```python
from build123d import *

# Parameters (mm, degrees)
F0_W        = 98
F0_H        = 136
F0_W_2      = 78
F0_H_2      = 116
F0_W_3      = 75
F0_H_3      = 113
F1_DEPTH    = 5
F2_W        = 78
F2_H        = 130
F3_DEPTH    = 0.5
F5_T1_DEPTH = 85
F6_R        = 5


# Not quite as in the source:
# - a fillet or chamfer that OpenCascade refuses, or shapes differently, is made with other operations: its cross-section is extruded or revolved along the edge and cut away or added
# - a feature of the source that left no trace in its solid (it failed there, or was rolled back) is left out


with BuildPart() as f1:
    # F0 (on Top) → F1 (new body, symmetric)
    with BuildSketch(Plane.XY):
        Rectangle(F0_W, F0_H)
        Rectangle(F0_W_2, F0_H_2, mode=Mode.SUBTRACT)
        Rectangle(F0_W_2, F0_H_2)
        Rectangle(F0_W_3, F0_H_3, mode=Mode.SUBTRACT)
    extrude(amount=F1_DEPTH, both=True)

    # F2 (on Top) → F3 (cut, symmetric)
    with BuildSketch(Plane.XY):
        with Locations((0, 7)):
            Rectangle(F2_W, F2_H)
    extrude(amount=F3_DEPTH, both=True, mode=Mode.SUBTRACT)

    # F5: fillet of radius 15 on 4 edges, made by hand

    # F5_s2 → F5_t1 (cut)
    with BuildSketch(Plane.XY.offset(-42.5)):
        with BuildLine():
            ThreePointArc((-34, -68), (-44.6066017178, -63.6066017178), (-49, -53))
            Line((-49, -53), (-49, -68))
            Line((-49, -68), (-34, -68))
        make_face()
        with BuildLine():
            ThreePointArc((34, -68), (44.6066017178, -63.6066017178), (49, -53))
            Line((49, -53), (49, -68))
            Line((49, -68), (34, -68))
        make_face()
        with BuildLine():
            ThreePointArc((34, 68), (44.6066017178, 63.6066017178), (49, 53))
            Line((49, 53), (49, 68))
            Line((49, 68), (34, 68))
        make_face()
        with BuildLine():
            ThreePointArc((-34, 68), (-44.6066017178, 63.6066017178), (-49, 53))
            Line((-49, 53), (-49, 68))
            Line((-49, 68), (-34, 68))
        make_face()
    extrude(amount=F5_T1_DEPTH, mode=Mode.SUBTRACT)

    # F6
    f6_edges = [f1.edges().sort_by_distance(p)[0] for p in [
        (37.5, -56.5, -2.75),
        (37.5, -56.5, 2.75),
        (-37.5, -56.5, 2.75),
        (-37.5, -56.5, -2.75),
        (-37.5, 56.5, 2.75),
        (-37.5, 56.5, -2.75),
        (37.5, 56.5, -2.75),
        (37.5, 56.5, 2.75),
    ]]
    fillet(f6_edges, radius=F6_R)


solid = f1.part
```
Check sheet for the modelled part. Datum: model origin and axes. Units: mm. A direction names the side the tool comes from. Coordinates: 2 decimals unless noted, no trailing zeros. Order: outer loops, then holes, each group sorted by start corner. A loop starts at its lowest first (then second) coordinate and runs counter-clockwise, first axis right, second up. Notation, with made-up numbers: (42, 47.25) -> (69, 47.25) arc R5 ccw to (69, 54.25) -> close; hole circle Ø1 at (17, -22). An arc over 180 degrees is marked (long way). Write each question's results on one line, items separated by ' | '. Start each with the question number.
1) Depth check by flat-ended pin: pin 1 (8 mm diameter, centred on x = 35.5, y = -9.5, fed in from -Z); pin 2 (0.8 mm diameter, centred on x = 3.5, z = 0, fed in from +Y). Enter the tip coordinate at first touch or a pass-through.
2) Set-up check for faces 1 (the face through (49, -1, 0)), 2 (the face through (37.5, -1, 3)): record each of +Z, -Z, +X, -X, +Y, -Y from which the full face is reachable in a straight line by a thin tool's end or side.
3) Draft check along Y on faces 3 (the face through (36.07, 55, -2.78)), 4 (the face through (0, 68, -3)), 5 (the face through (-9, 57, -0.5)). Enter one of: pulls with the +Y half, pulls with the -Y half, needs draft (parallel to the pull), parting line crosses it, or undercut.
4) Section check B-B (y = 38). Enter the section's corners in (x, z), and give its area (3 significant figures).
5) Section check C-C (z = 3.25). Enter the section's corners in (x, y), and give its area (3 significant figures).
6) Material ranges on line 1 along X through (y, z) = (-25, 2); line 2 along Y through (x, z) = (21, 2.25); line 3 along Z through (x, y) = (-38, 35), recorded low to high.
7) Section check A-A (x = -3.5). Enter the section's corners in (y, z), and give its area (3 significant figures).
Checked values:
1) pin 1: z = -5 | pin 2: y = -58
2) face 1: +Z, -Z, +X, +Y, -Y | face 2: +Z, -Z
3) face 3: undercut | face 4: pulls with the +Y half | face 5: needs draft
4) outline: (-49, -5) -> (-37.5, -5) -> (-37.5, -0.5) -> (-39, -0.5) -> (-39, 0.5) -> (-37.5, 0.5) -> (-37.5, 5) -> (-49, 5) -> close; (37.5, -5) -> (49, -5) -> (49, 5) -> (37.5, 5) -> (37.5, 0.5) -> (39, 0.5) -> (39, -0.5) -> (37.5, -0.5) -> close | area: 227 mm²
5) outline: (-49, -53) arc R15 ccw to (-34, -68) -> (34, -68) arc R15 ccw to (49, -53) -> (49, 53) arc R15 ccw to (34, 68) -> (-34, 68) arc R15 ccw to (-49, 53) -> close; hole (-37.5, -51.5) arc R5 ccw to (-32.5, -56.5) -> (32.5, -56.5) arc R5 ccw to (37.5, -51.5) -> (37.5, 51.5) arc R5 ccw to (32.5, 56.5) -> (-32.5, 56.5) arc R5 ccw to (-37.5, 51.5) -> close | area: 4,680 mm²
6) line 1: -49 to -37.5, 37.5 to 49 | line 2: -68 to -56.5, 56.5 to 68 | line 3: -5 to -0.5, 0.5 to 5
7) outline: (-68, -5) -> (-56.5, -5) -> (-56.5, -0.5) -> (-58, -0.5) -> (-58, 0.5) -> (-56.5, 0.5) -> (-56.5, 5) -> (-68, 5) -> close; (56.5, -5) -> (68, -5) -> (68, -0.5) -> (56.5, -0.5) -> close; (56.5, 0.5) -> (68, 0.5) -> (68, 5) -> (56.5, 5) -> close | area: 217 mm²
